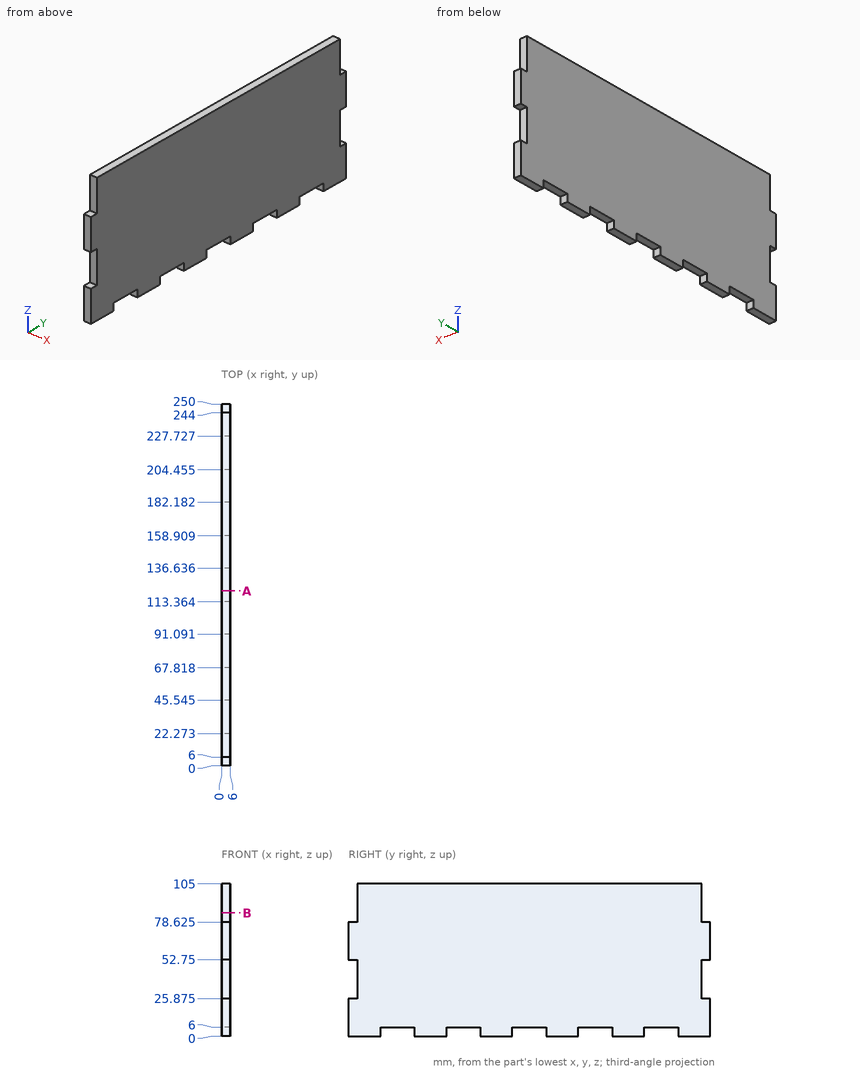
Check sheet for the drawn part. Datum: minimum x, y, z corner. Units: mm. Round coordinates to 2 decimals unless told otherwise and drop trailing zeros. Write each loop counter-clockwise with the first axis right and the second up, starting at its lowest first coordinate (ties: lowest second). Pieces come first, ordered by that corner, then holes. Notation, with made-up numbers: (5.5, 23.25) -> (11.5, 23.25) arc R33 cw to (11.5, 53.25) -> close; hole circle Ø9 at (79.5, 83.5). An arc over 180 degrees is marked (long way). One line per item, written item: value. Start each with the question number.
(1) Scan lines: line 1 (Z direction, x = 3.2, y = 120.5); line 2 (Y direction, x = 2.5, z = 93.5). Record each from-to range of solid material in increasing order. Write a range as [from, to].
(2) Cross-section at B-B, the plane z = 85. Record the cut outline in (x, y).
(3) Cross-section at A-A, the plane y = 121. Record the cut outline in (x, z), and give its area (3 significant figures).
(4) Go/stop test with flat-tipped pins: pin 1 Ø1.8 at (x, y) = (4.5, 121.5) entering from -Z; pin 2 Ø3 at (x, z) = (3.5, 44) entering from +Y. Record where each tip stops, or that it passes through.
Answer:
1. line 1: [6, 105]
1. line 2: [6, 244]
2. outline: (0, 6) -> (6, 6) -> (6, 244) -> (0, 244) -> close
3. outline: (0, 6) -> (6, 6) -> (6, 105) -> (0, 105) -> close
3. area: 594 mm²
4. pin 1: z = 6
4. pin 2: y = 244
